Autodesk Inventor part; units mm, degrees
ref_plane "XZ Plane" through (0, 0, 0) normal (0, 1, 0) x (-1, 0, 0)
sketch "Sketch1" plane through (0, 0, 0) normal (0, 1, 0) x (-1, 0, 0)
  line L0 (-12, 14) -> (12, 14) construction
  line L1 (14, 12) -> (14, -12) construction
  line L2 (12, -14) -> (-12, -14) construction
  line L3 (-14, -12) -> (-14, 12) construction
  line L4 (-14, 14) -> (14, -14) construction
  line L5 (14, 14) -> (-14, -14) construction
  arc A0 (14, 12) -> (12, 14) centre (12, 12) ccw construction
  arc A1 (12, -14) -> (14, -12) centre (12, -12) ccw construction
  arc A2 (-14, -12) -> (-12, -14) centre (-12, -12) ccw construction
  arc A3 (-12, 14) -> (-14, 12) centre (-12, 12) ccw construction
  line L6 (-12, -15) -> (12, -15)
  arc A4 (12, -15) -> (15, -12) centre (12, -12) ccw
  line L7 (15, -12) -> (15, 12)
  arc A5 (15, 12) -> (12, 15) centre (12, 12) ccw
  line L8 (12, 15) -> (-12, 15)
  arc A6 (-12, 15) -> (-15, 12) centre (-12, 12) ccw
  line L9 (-15, 12) -> (-15, -12)
  arc A7 (-15, -12) -> (-12, -15) centre (-12, -12) ccw
  line L10 (13, -12) -> (13, 12)
  arc A8 (13, 12) -> (12, 13) centre (12, 12) ccw
  line L11 (12, 13) -> (-12, 13)
  arc A9 (-12, 13) -> (-13, 12) centre (-12, 12) ccw
  line L12 (-13, 12) -> (-13, -12)
  arc A10 (-13, -12) -> (-12, -13) centre (-12, -12) ccw
  line L13 (-12, -13) -> (12, -13)
  arc A11 (12, -13) -> (13, -12) centre (12, -12) ccw
  point P0 (0, 0)
  point P1 (0, 0)
  point P2 (0, 0)
  dimension "d10" = 2
  dimension "depth" = 30
  dimension "width" = 30
  dimension "thickness" = 2
extrude "Extrusion1" add sketch "Sketch1" along normal blind 500
sketch "Sketch2" plane through (12, 0, -15) normal (0, 0, -1) x (-1, 0, 0)
  line L0 (12, -470) -> (12, 2820) construction
  line L1 (0, 0) -> (24, 0)
  point P0 (12, 0)
  point P1 (12, 50)
  point P2 (12, 100)
  dimension "d16" = 50
  dimension "d17" = 50
hole "Hole1" at (0, 50, -15) at (0, 100, -15) direction (0, 0, 1) diameter 9 depth 20.2 tip angle 118
sketch "Sketch3" plane through (12, 0, -15) normal (0, 0, -1) x (-1, 0, 0)
  line L0 (12, -100) -> (12, 600) construction
  circle A0 centre (-588, 1200) radius 1000
  point P0 (12, 0)
  dimension "d29" = 2000
  dimension "d31" = 1200
  dimension "d34" = 600
extrude "Extrusion2" cut sketch "Sketch3" against normal through all
equation "\"d10\" = thickness"
properties part number "noga do okraglej duzej P" material "Steel"
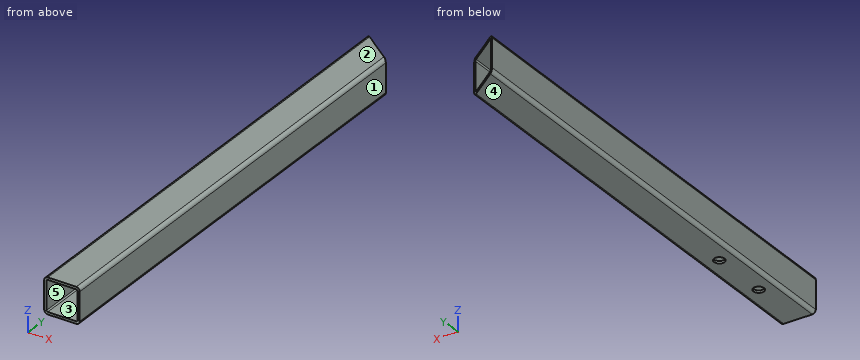
For this review, take the finished solid that the model builds, in its own axes (mm). Face numbers are marked on the shaded views. A direction names the side the tool comes from. Coordinates: 2 decimals unless noted, no trailing zeros. Loops run counter-clockwise (first coordinate to the right, second up) from the corner with the lowest first, then second, coordinate; pieces in that order, holes last. Notation, with made-up numbers: (28.5, 10.5) -> (75.5, 10.5) arc R32 cw to (75.5, 46.5) -> close; hole circle Ø5 at (-26, 44). An arc over 180 degrees is marked (long way). Return JSON: item names as keys, results as strings. Group by question number.
(1) Consider section B-B, the plane x = 0. Give the boundary of the cut face in (y, z), plus the area to 3 significant figures.
(2) Tool access review of the marked faces 4 and 5: name each direction out of +Z, -Z, +X, -X, +Y, -Y from which nothing blocks a thin tool from reaching the whole face with its end or side.
(3) To check wall thickness, follow L1, parallel to Z at x = -1.5, y = 203.5; L2, parallel to Y at x = 0, z = -13.6. State the ranges of each line that lie inside material, in increasing order.
(4) Consider section A-A, the plane z = -7. Give the boundary of the cut face in (x, y), plus the area to 3 significant figures.
(5) Consider section C-C, the plane y = 334. Give the boundary of the cut face in (x, z), plus the area to 3 significant figures.
(6) Mouldability with a two-part tool opening along Z and no side actions: class the marked faces 1, 2 and 3 as pulls with the +Z half, pulls with the -Z half, needs draft (parallel to the pull), parting line crosses it, or undercut.
(7) Consider section D-D, the plane y = 50. Give the boundary of the cut face in (x, z), plus the area to 3 significant figures.
(8) For pin 1 Ø5.5 at (x, y) = (0, 50) entering from -Z, flat-tipped, find the tip position at first contact; note if it passes through.
Results below:
{
 "1": {"outline": "(0, -15) -> (45.5, -15) -> (45.5, -13) -> (0, -13) -> close; (0, 13) -> (400, 13) -> (400, 15) -> (0, 15) -> close; (54.5, -15) -> (95.5, -15) -> (95.5, -13) -> (54.5, -13) -> close; (104.5, -15) -> (400, -15) -> (400, -13) -> (104.5, -13) -> close", "area": "1,560 mm2"},
 "2": {"face 4": "-Z, +X, -X, +Y, -Y", "face 5": "+Y, -Y"},
 "3": {"L1": "z = -15 to -13, 13 to 15", "L2": "y = 0 to 45.5, 54.5 to 95.5, 104.5 to 400"},
 "4": {"outline": "(-15, 0) -> (-13, 0) -> (-13, 409.92) arc R1000 cw to (-15, 411.47) -> close; (13, 0) -> (15, 0) -> (15, 388.97) arc R1000 cw to (13, 390.41) -> close", "area": "1,600 mm2"},
 "5": {"outline": "(-15, -12) arc R3 ccw to (-12, -15) -> (12, -15) arc R3 ccw to (15, -12) -> (15, 12) arc R3 ccw to (12, 15) -> (-12, 15) arc R3 ccw to (-15, 12) -> close; hole (-13, -12) arc R1 ccw to (-12, -13) -> (12, -13) arc R1 ccw to (13, -12) -> (13, 12) arc R1 ccw to (12, 13) -> (-12, 13) arc R1 ccw to (-13, 12) -> close", "area": "217 mm2"},
 "6": {"face 1": "needs draft", "face 2": "pulls with the +Z half", "face 3": "undercut"},
 "7": {"outline": "(-15, -12) arc R3 ccw to (-12, -15) -> (-4.5, -15) -> (-4.5, -13) -> (-12, -13) arc R1 cw to (-13, -12) -> (-13, 12) arc R1 cw to (-12, 13) -> (12, 13) arc R1 cw to (13, 12) -> (13, -12) arc R1 cw to (12, -13) -> (4.5, -13) -> (4.5, -15) -> (12, -15) arc R3 ccw to (15, -12) -> (15, 12) arc R3 ccw to (12, 15) -> (-12, 15) arc R3 ccw to (-15, 12) -> close", "area": "199 mm2"},
 "8": {"pin 1": "stops at z = 13"}
}
